Input: part model. Units: mm. Frame: model coordinates. A direction names the side the tool comes from. Give positions to 0.01 mm unless a question says otherwise; leave off trailing zeros. Loops run counter-clockwise (first coordinate to the right, second up) from the corner with the lowest first, then second, coordinate; pieces in that order, holes last.
from build123d import *

# Parameters (mm, degrees)
F3_DEPTH      = 25
F3_DEPTH_BACK = 25
F7_R          = 3.75
F8_DEPTH      = 175.008284


with BuildPart() as f3:
    # F1 (on Front) → F3 (new body, two sides)
    with BuildSketch(Plane.XZ) as f3_sk:
        Polygon((-13.689034, 164.416686), (-18.182479, 170.359462), (-18.182479, 166.913599), (-14.472469, 162.748992), (-8.156137, 158.776864), (5.172722, 144.838229), (-4.562378, 133.733749), (-6.996153, 125.563219), (-12.993669, 118.435733), (-18.100433, 108.785093), (-18.182479, 104.653799), (-12.05458, 117.461517), (-6.668613, 123.716192), (3.25861, 104.569836), (10.598217, 100.251484), (3.565824, 93.206773), (-7.237375, 74.845315), (-18.281374, 68.406361), (-18.237878, 66.536016), (-6.20943, 73.651383), (-4.18945, 77.084604), (8.558222, 65.844081), (18.144256, 51.864788), (18.144256, 54.47248), (9.574368, 66.883489), (-3.439697, 78.358909), (4.734092, 92.251338), (11.93507, 99.464929), (18.187713, 95.84786), (18.187713, 97.673245), (4.161306, 105.989113), (-5.645856, 124.90391), (-3.268425, 132.966489), (6.69481, 144.126818), (13.16941, 141.100645), (18.144252, 131.225541), (18.144252, 135.615155), (14.830102, 142.302305), (6.104447, 146.795377), (-7.517676, 160.505265), (4.814246, 169.316471), (7.670024, 174.035177), (5.975025, 174.078628), (3.461061, 170.081015), (-8.945923, 161.410491), align=None)
    extrude(amount=F3_DEPTH)
    extrude(f3_sk.sketch, amount=-F3_DEPTH_BACK)

    # F4 (on Front) → F5 (revolve, cut)
    with BuildSketch(Plane.XZ):
        Polygon((50.79839, 174.967825), (17.925017, 175.093472), (17.925017, -3.259191), (50.79839, -3.259191), align=None)
    revolve(axis=Axis((0, 0, 87.499648), (0, 0, 1)), mode=Mode.SUBTRACT)

    # F2 (on Front) → F6 (revolve)
    with BuildSketch(Plane.XZ):
        Polygon((-3.515409, 175.007284), (-20.104863, 174.987718), (-20.104863, 0), (-9.95, 0), (-9.95, 25.057623), (-15.821613, 33.821163), (-15.821613, 71.417056), (-17.904863, 100.988127), (-17.904863, 173.787653), (-3.515409, 173.787653), align=None)
    revolve(axis=Axis((0, 0, 12.804373), (0, 0, 1)))

    # F7 (on face) → F8 (cut, through all)
    with BuildSketch(Plane(origin=(0, 0, 0), x_dir=(1, 0, 0), z_dir=(0, 0, -1))):
        Circle(F7_R)
    extrude(amount=-F8_DEPTH, mode=Mode.SUBTRACT)


solid = f3.part
(1) Pin query (flat end, axial travel): pin 1 Ø12 at (y, z) = (13.5, 114.5) entering from +X; pin 2 Ø1 at (y, z) = (3.5, 92.5) entering from +X; pin 3 Ø8 at (x, z) = (3.5, 63) entering from +Y. Return the tip coordinate at first contact, or that it passes through.
Values follow:
pin 1: stops at x = 18.65
pin 2: stops at x = 19.88
pin 3: stops at y = 20.1
(2) Reachability of faces 1 (the flat face through (-11.36, -0.22, 160.79)), 2 (the cylindrical face through (-3.746, -0.165, 174.389)) from +Z, -Z, +X, -X, +Y, -Y: full face, straight path, thin tool, end or side. Return the list, or none.
Values follow:
face 1: none
face 2: +Z, -Z
(3) Ray query, probe 1 along X at (y, z) = (0, 135); probe 2 along Z at (x, y) = (12, 1); probe 3 along Y at (x, z) = (0, 150). Return the intervals inside material, ascending.
Values follow:
probe 1: x = -20.1 to -17.9, 16.24 to 20.1
probe 2: z = 0 to 28.18, 60.82 to 63.37, 99.43 to 101.34, 141.65 to 143.76, 173.79 to 175
probe 3: y = -20.1 to -17.9, 17.9 to 20.1
(4) Cut plane B-B (y = -6). Count the separate pieces of the cut face and the enclosed holes in it, and give its area (3 significant figures).
Values follow:
separate pieces: 1
enclosed holes: 6
area: 1,970 mm2
(5) Cut plane C-C (z = 37). Return the cut outline in (x, y), and give its area (3 significant figures).
Values follow:
outline: circle Ø40.21 at (0, 0); hole circle Ø31.64 at (0, 0)
area: 483 mm2
